from build123d import *

# Parameters (mm, degrees)
SKETCH_1_W             = 48
SKETCH_1_H             = 48
SKETCH_1_R             = 16.8
SKETCH_1_R_2           = 1.67
EXTRUDE_1_DEPTH        = 21.5
SKETCH_3_W             = 60
SKETCH_3_H             = 48
SKETCH_3_R             = 2.15
EXTRUDE_2_DEPTH        = 18
PATTERN_LINEAR_2_COUNT = 2
PATTERN_LINEAR_2_PITCH = 108


with BuildPart() as part:
    # 草图1 → 凸台-拉伸1 (new body)
    with BuildSketch(Plane.XY):
        Rectangle(SKETCH_1_W, SKETCH_1_H)
        Circle(SKETCH_1_R, mode=Mode.SUBTRACT)
        with Locations((-19, 19)):
            Circle(SKETCH_1_R_2, mode=Mode.SUBTRACT)
        with Locations((19, 19)):
            Circle(SKETCH_1_R_2, mode=Mode.SUBTRACT)
        with Locations((19, -19)):
            Circle(SKETCH_1_R_2, mode=Mode.SUBTRACT)
        with Locations((-19, -19)):
            Circle(SKETCH_1_R_2, mode=Mode.SUBTRACT)
    extrude_1 = extrude(amount=EXTRUDE_1_DEPTH)

    # 草图3 → 凸台-拉伸2 (add)
    with BuildSketch(Plane.XY.offset(21.5)):
        with Locations((54, 0)):
            Rectangle(SKETCH_3_W, SKETCH_3_H)
        with Locations((54, 17)):
            Circle(SKETCH_3_R, mode=Mode.SUBTRACT)
        with Locations((54, 0)):
            Circle(SKETCH_3_R, mode=Mode.SUBTRACT)
        with Locations((54, -17)):
            Circle(SKETCH_3_R, mode=Mode.SUBTRACT)
    extrude(amount=-EXTRUDE_2_DEPTH)

    # 阵列(线性)2: 凸台-拉伸1 ×2
    with Locations(*[(i * PATTERN_LINEAR_2_PITCH, 0, 0) for i in range(1, PATTERN_LINEAR_2_COUNT)]):
        add(extrude_1)


solid = part.part
Could you check a few things on this model? Use its own coordinates, in mm. A direction names the side the tool comes from. Give positions to 0.01 mm unless a question says otherwise; leave off trailing zeros. Order: outer loops, then holes, each group sorted by start corner. A loop starts at its lowest first (then second) coordinate and runs counter-clockwise, first axis right, second up. Notation, with made-up numbers: (42, -21.5) -> (57, -21.5) arc R21 ccw to (57, -13.5) -> close; hole circle Ø1 at (13.5, -39.75). An arc over 180 degrees is marked (long way). Return JSON: item names as keys, results as strings.
1. I need wall thicknesses on line 1 (Y direction, x = 127, z = 12.5); line 2 (Y direction, x = 54, z = 8); line 3 (Y direction, x = 0, z = 7.25). Which ranges of each line are inside material? Lowest first, please. Write a range as from..to.
Answer list:
{"line 1": "y = -24..-20.67, -17.33..17.33, 20.67..24", "line 2": "y = -24..-19.15, -14.85..-2.15, 2.15..14.85, 19.15..24", "line 3": "y = -24..-16.8, 16.8..24"}
2. On a 3-axis mill with a long thin cutter (end or side, diameter ignored), from which of +Z, -Z, +X, -X, +Y, -Y can I reach the whole of each face in a straight line? I mean faces 1 (the cylindrical face through (128.543, -19.64, 10.599)), 2 (the flat face through (84, 0, 2)). Say none if no direction works.
Answer list:
{"face 1": "+Z, -Z", "face 2": "-Z, +Y, -Y"}
3. Imagine slicing it at B-B on x = 89. List the corners of the cut face in (y, z) for me.
Answer list:
{"outline": "(-24, 0) -> (-20.67, 0) -> (-20.67, 21.5) -> (-24, 21.5) -> close; (-17.33, 0) -> (17.33, 0) -> (17.33, 21.5) -> (-17.33, 21.5) -> close; (20.67, 0) -> (24, 0) -> (24, 21.5) -> (20.67, 21.5) -> close"}
4. Thinking about a two-plate mould opening in X: for faces 3 (the flat face through (53, -24, 11)), 4 (the flat face through (132, 0, 11)), 5 (the cylindrical face through (91.216, 0.739, 10.599)), which applies, pulls with the +X half, pulls with the -X half, needs draft (parallel to the pull), parting line crosses it, or undercut?
Answer list:
{"face 3": "needs draft", "face 4": "pulls with the +X half", "face 5": "undercut"}
5. Imagine slicing it at D-D on z = 11.25. Give the number of separate pieces and of enclosed holes in the cut face, then the cut area to 3 significant figures.
Answer list:
{"separate pieces": "1", "enclosed holes": "13", "area": "5,600 mm2"}
6. Imagine slicing it at C-C on y = -4.5. List the corners of the cut face in (x, z) for me, then the cut area to 3 significant figures.
Answer list:
{"outline": "(-24, 0) -> (-16.19, 0) -> (-16.19, 21.5) -> (-24, 21.5) -> close; (16.19, 0) -> (24, 0) -> (24, 3.5) -> (84, 3.5) -> (84, 0) -> (91.81, 0) -> (91.81, 21.5) -> (16.19, 21.5) -> close; (124.19, 0) -> (132, 0) -> (132, 21.5) -> (124.19, 21.5) -> close", "area": "1,750 mm2"}
7. Imagine slicing it at A-A on x = 54. List the corners of the cut face in (y, z) for me, then the cut area to 3 significant figures.
Answer list:
{"outline": "(-24, 3.5) -> (-19.15, 3.5) -> (-19.15, 21.5) -> (-24, 21.5) -> close; (-14.85, 3.5) -> (-2.15, 3.5) -> (-2.15, 21.5) -> (-14.85, 21.5) -> close; (2.15, 3.5) -> (14.85, 3.5) -> (14.85, 21.5) -> (2.15, 21.5) -> close; (19.15, 3.5) -> (24, 3.5) -> (24, 21.5) -> (19.15, 21.5) -> close", "area": "632 mm2"}
8. For pin 1 Ø3.5 at (x, y) = (54, 17) entering from +Z, with a flat end and sliding along its axis, tell me the tip position at first contact or that it passes through.
Answer list:
{"pin 1": "passes through"}
